The model under review builds one solid part; all positions refer to its coordinate system, in mm. A direction names the side the tool comes from. Coordinates: 2 decimals unless noted, no trailing zeros. Write each loop counter-clockwise with the first axis right and the second up, starting at its lowest first coordinate (ties: lowest second). Pieces come first, ordered by that corner, then holes. Notation, with made-up numbers: (-21.75, -39) - (24.25, -39) arc R25 cw to (24.25, -16) - close; hole circle Ø9 at (51.5, -9.5). An arc over 180 degrees is marked (long way). Use one line per item in the form item = value. Start each with the question number.
```python
from build123d import *

# Parameters (mm, degrees)
SKETCH1_R           = 17.5
BOSS_EXTRUDE1_DEPTH = 35
CUT_EXTRUDE1_DEPTH  = 15
SKETCH3_R           = 4.1
CUT_EXTRUDE2_DEPTH  = 32.819805153
SKETCH4_R           = 2
CUT_EXTRUDE3_DEPTH  = 43.866070499
SKETCH5_R           = 14.5
CUT_EXTRUDE4_DEPTH  = 5


with BuildPart() as part:
    # Sketch1 → Boss-Extrude1 (new body)
    with BuildSketch(Plane(origin=(0, 0, 0), x_dir=(1, 0, 0), z_dir=(0, 1, 0))):
        with Locations(Location((0, 0, 0), (0, 0, 270))):
            Circle(SKETCH1_R)
    extrude(amount=BOSS_EXTRUDE1_DEPTH)

    # Sketch2 → Cut-Extrude1 (cut)
    with BuildSketch(Plane(origin=(0, 35, 0), x_dir=(1, 0, 0), z_dir=(0, 1, 0))):
        Polygon((0, 7.7), (-6.668395609, 3.85), (-6.668395609, -3.85), (0, -7.7), (6.668395609, -3.85), (6.668395609, 3.85), align=None)
    extrude(amount=-CUT_EXTRUDE1_DEPTH, mode=Mode.SUBTRACT)

    # Sketch3 → Cut-Extrude2 (cut, through all)
    with BuildSketch(Plane(origin=(0, 20, 0), x_dir=(1, 0, 0), z_dir=(0, 1, 0))):
        with Locations(Location((0, 0, 0), (0, 0, 270))):
            Circle(SKETCH3_R)
    extrude(amount=-CUT_EXTRUDE2_DEPTH, mode=Mode.SUBTRACT)

    # Sketch4 → Cut-Extrude3 (cut, through all)
    with BuildSketch(Plane(origin=(0, 35, 0), x_dir=(1, 0, 0), z_dir=(0, 1, 0))):
        with Locations(Location((-9, 9, 0), (0, 0, 270))):
            Circle(SKETCH4_R)
        with Locations(Location((9, 9, 0), (0, 0, 270))):
            Circle(SKETCH4_R)
        with Locations(Location((9, -9, 0), (0, 0, 270))):
            Circle(SKETCH4_R)
        with Locations(Location((-9, -9, 0), (0, 0, 270))):
            Circle(SKETCH4_R)
    extrude(amount=-CUT_EXTRUDE3_DEPTH, mode=Mode.SUBTRACT)

    # Sketch5 → Cut-Extrude4 (cut)
    with BuildSketch(Plane(origin=(0, 35, 0), x_dir=(1, 0, 0), z_dir=(0, 1, 0))):
        Circle(SKETCH5_R)
    extrude(amount=-CUT_EXTRUDE4_DEPTH, mode=Mode.SUBTRACT)


solid = part.part
```
1. The part is to be moulded in two halves that separate along Z. For faces 1 (the flat face through (13, 35, -7)), 2 (the flat face through (-6.668, 25, 0)), 3 (the cylindrical face through (-10.648, 17.255, -13.887)), say which applies: released by +Z, released by -Z, zero draft, split by the parting line, or undercut.
2. Take a section at D-D (y = 31.5). State the section outline as (x, z) points.
3. For L1, parallel to X at y = 28, z = 0.5; L2, parallel to Z at x = -9, y = 14; L3, parallel to X at y = 25, z = -8.5, list the stretches that pass through material, from the lowest coordinate up.
4. For P1, Ø2.5, axis at x = -9, z = -9, coming from the -Y side; P2, Ø12, axis at x = 8.5, y = 24, coming from the +Z side; P3, Ø14.5, axis at x = -0.5, z = -0.5, coming from the +Y side; P4, Ø6, axis at x = -9, y = 8.5, coming from the +Z side, all flat-tipped, find the tip position at first contact; note any pin that passes through.
5. Take a section at C-C (z = 3). State the section outline as (x, y) points, plus the area to 3 significant figures.
6. For faces 4 (the cylindrical face through (4.065, 10.14, -0.534)), 5 (the flat face through (-3.38, 25.07, 5.75)), list the 3-axis set-ups (+Z, -Z, +X, -X, +Y, -Y) from which the entire face can be reached by the end or side of a thin tool; tool diameter is ignored.
7. Take a section at A-A (y = 24). State the section outline as (x, z) points, plus the area to 3 significant figures.
8. Take a section at B-B (x = -9). State the section outline as (y, z) points, plus the area to 3 significant figures.
Returned:
q1.face_1 = zero draft
q1.face_2 = undercut
q1.face_3 = split by the parting line
q2.outline = circle Ø35 at (0, 0); hole (-10.93, -9.53) arc R2 ccw to (-9.53, -10.93) arc R14.5 ccw to (9.53, -10.93) arc R2 ccw to (10.93, -9.53) arc R14.5 ccw to (10.93, 9.53) arc R2 ccw to (9.53, 10.93) arc R14.5 ccw to (-9.53, 10.93) arc R2 ccw to (-10.93, 9.53) arc R14.5 ccw to start
q3.L1 = -17.49 to -6.67, 6.67 to 17.49
q3.L2 = -15.01 to -11, -7 to 7, 11 to 15.01
q3.L3 = -15.3 to -10.94, -7.06 to 7.06, 10.94 to 15.3
q4.P1 = through
q4.P2 = 17.32
q4.P3 = 30
q4.P4 = 16.44
q5.outline = (-17.24, 0) - (-2.79, 0) - (-2.79, 20) - (-6.67, 20) - (-6.67, 30) - (-14.19, 30) - (-14.19, 35) - (-17.24, 35) - close; (2.79, 0) - (17.24, 0) - (17.24, 35) - (14.19, 35) - (14.19, 30) - (6.67, 30) - (6.67, 20) - (2.79, 20) - close
q5.area = 820 mm²
q6.face_4 = +Y, -Y
q6.face_5 = +Y
q7.outline = circle Ø35 at (0, 0); hole circle Ø4 at (-9, -9); hole circle Ø4 at (-9, 9); hole (-6.67, -3.85) - (0, -7.7) - (6.67, -3.85) - (6.67, 3.85) - (0, 7.7) - (-6.67, 3.85) - close; hole circle Ø4 at (9, -9); hole circle Ø4 at (9, 9)
q7.area = 758 mm²
q8.outline = (0, -15.01) - (35, -15.01) - (35, -11.37) - (30, -11.37) - (30, -11) - (0, -11) - close; (0, -7) - (30, -7) - (30, 7) - (0, 7) - close; (0, 11) - (30, 11) - (30, 11.37) - (35, 11.37) - (35, 15.01) - (0, 15.01) - close
q8.area = 697 mm²
